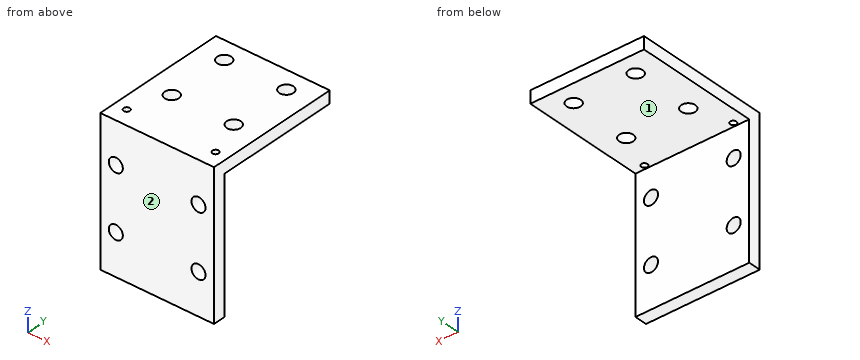
from build123d import *

# Parameters (mm, degrees)
SKETCH1_W                = 27.5
SKETCH1_H                = 3
BOSS_EXTRUDE1_DEPTH      = 35
SKETCH2_W                = 27.5
SKETCH2_H                = 3
BOSS_EXTRUDE2_DEPTH      = 40
M3_CLEARANCE_HOLE1_D     = 3.4
M3_CLEARANCE_HOLE1_DEPTH = 5
M3_CLEARANCE_HOLE1_TIP   = 1.021463052
SKETCH6_R                = 0.75
CUT_EXTRUDE1_DEPTH       = 10
M3_CLEARANCE_HOLE2_D     = 3.4
M3_CLEARANCE_HOLE2_DEPTH = 5
M3_CLEARANCE_HOLE2_TIP   = 1.021463052
SKETCH12_W               = 27.5
SKETCH12_H               = 10
CUT_EXTRUDE2_DEPTH       = 4


with BuildPart() as part:
    # Sketch1 → Boss-Extrude1 (new body)
    with BuildSketch(Plane.XY):
        Rectangle(SKETCH1_W, SKETCH1_H)
    extrude(amount=BOSS_EXTRUDE1_DEPTH)

    # Sketch2 → Boss-Extrude2 (add)
    with BuildSketch(Plane(origin=(0, 1.5, 0), x_dir=(1, 0, 0), z_dir=(0, 1, 0))):
        with Locations((0, -33.5)):
            Rectangle(SKETCH2_W, SKETCH2_H)
    extrude(amount=BOSS_EXTRUDE2_DEPTH)

    # M3 Clearance Hole1
    with Locations(Plane(origin=(0, 1.5, 0), x_dir=(1, 0, 0), z_dir=(0, 1, 0))):
        with Locations((-10, -10), (-10, -25), (10, -25), (10, -10)):
            Hole(M3_CLEARANCE_HOLE1_D / 2, depth=M3_CLEARANCE_HOLE1_DEPTH)
            with Locations((0, 0, -(M3_CLEARANCE_HOLE1_DEPTH + M3_CLEARANCE_HOLE1_TIP / 2))):  # 118° drill point
                Cone(0, M3_CLEARANCE_HOLE1_D / 2, M3_CLEARANCE_HOLE1_TIP, mode=Mode.SUBTRACT)

    # Sketch6 → Cut-Extrude1 (cut)
    with BuildSketch(Plane.XY.offset(35)):
        with Locations((-10.75, 2.5)):
            Circle(SKETCH6_R)
    cut_extrude1 = extrude(amount=-CUT_EXTRUDE1_DEPTH, mode=Mode.SUBTRACT)

    # M3 Clearance Hole2
    with Locations(Plane(origin=(0, 0, 32), x_dir=(-1, 0, 0), z_dir=(0, 0, -1))):
        with Locations((-7.5, 11.5), (7.5, 11.5), (7.5, 26.5), (-7.5, 26.5)):
            Hole(M3_CLEARANCE_HOLE2_D / 2, depth=M3_CLEARANCE_HOLE2_DEPTH)
            with Locations((0, 0, -(M3_CLEARANCE_HOLE2_DEPTH + M3_CLEARANCE_HOLE2_TIP / 2))):  # 118° drill point
                Cone(0, M3_CLEARANCE_HOLE2_D / 2, M3_CLEARANCE_HOLE2_TIP, mode=Mode.SUBTRACT)

    # Mirror1: Cut-Extrude1 across plane
    add(cut_extrude1.mirror(Plane(origin=(0, 0, 0), x_dir=(0, 0, 1), z_dir=(1, 0, 0))), mode=Mode.SUBTRACT)

    # Sketch12 → Cut-Extrude2 (cut, through all)
    with BuildSketch(Plane(origin=(0, 0, 32), x_dir=(-1, 0, 0), z_dir=(0, 0, -1))):
        with Locations((0, 36.5)):
            Rectangle(SKETCH12_W, SKETCH12_H)
    extrude(amount=-CUT_EXTRUDE2_DEPTH, mode=Mode.SUBTRACT)


solid = part.part
Geometry: final body of the model. Coordinates: model frame, mm. Face numbers are marked on the shaded views. A direction names the side the tool comes from. Give positions to 0.01 mm unless a question says otherwise; leave off trailing zeros. Write each loop counter-clockwise with the first axis right and the second up, starting at its lowest first coordinate (ties: lowest second). Pieces come first, ordered by that corner, then holes. Notation, with made-up numbers: M 84,18.5 L 140,18.5 A10 ccw 140,36.5 Z; hole C 52,51.5 d10. An arc over 180 degrees is marked long. Answer in a Markdown table with one row per item. Add a question column.
(1) Ray query, line 1 (X direction, y = -0.15, z = 25); line 2 (Y direction, x = 10.75, z = 33.65); line 3 (X direction, y = 27, z = 33). Return the intervals inside material, ascending.
(2) Section A-A on x = -7.5. Return loops of the section in (y, z), and give its area (3 significant figures).
(3) Section B-B on y = 2.5. Return loops of the section in (x, z), and give its area (3 significant figures).
(4) First-contact query: pin 1 (4 mm diameter, centred on x = -10, z = 25, fed in from -Y); pin 2 (2.5 mm diameter, centred on x = 7.5, y = 11.5, fed in from +Z); pin 3 (5.5 mm diameter, centred on x = 10, z = 25, fed in from +Y); pin 4 (1.7 mm diameter, centred on x = -10.75, y = 2.5, fed in from -Z). Flat tips, straight axial feed; report the tip coordinate or a pass-through.
(5) Section D-D on x = -10.75. Return loops of the section in (y, z).
(6) Reachability of the marked faces 1 and 2 from +Z, -Z, +X, -X, +Y, -Y: full face, straight path, thin tool, end or side. Return the list, or none.
(7) Section C-C on z = 10. Return loops of the section in (x, y), and give its area (3 significant figures).
Result set:
| question | item | result |
|---|---|---|
| 1 | line 1 | x = -13.75 to -11.7, -8.3 to 8.3, 11.7 to 13.75 |
| 1 | line 2 | y = -1.5 to 1.75, 3.25 to 31.5 |
| 1 | line 3 | x = -13.75 to -9.12, -5.88 to 5.88, 9.12 to 13.75 |
| 2 | outline | M -1.5,0 L 1.5,0 L 1.5,32 L 9.8,32 L 9.8,35 L -1.5,35 Z; M 13.2,32 L 24.8,32 L 24.8,35 L 13.2,35 Z; M 28.2,32 L 31.5,32 L 31.5,35 L 28.2,35 Z |
| 2 | area | 175 mm^2 |
| 3 | outline | M -13.75,32 L -11.5,32 L -11.5,35 L -13.75,35 Z; M -10,32 L 10,32 L 10,35 L -10,35 Z; M 11.5,32 L 13.75,32 L 13.75,35 L 11.5,35 Z |
| 3 | area | 73.5 mm^2 |
| 4 | pin 1 | stops at y = -1.5 |
| 4 | pin 2 | passes through |
| 4 | pin 3 | stops at y = 1.5 |
| 4 | pin 4 | stops at z = 32 |
| 5 | outline | M -1.5,0 L 1.5,0 L 1.5,8.47 L -1.5,8.47 Z; M -1.5,11.53 L 1.5,11.53 L 1.5,23.47 L -1.5,23.47 Z; M -1.5,26.53 L 1.5,26.53 L 1.5,32 L 1.75,32 L 1.75,35 L -1.5,35 Z; M 3.25,32 L 31.5,32 L 31.5,35 L 3.25,35 Z |
| 6 | face 1 | -Z, +X, -X, +Y |
| 6 | face 2 | +Z, -Z, +X, -X, -Y |
| 7 | outline | M -13.75,-1.5 L -11.7,-1.5 L -11.7,1.5 L -13.75,1.5 Z; M -8.3,-1.5 L 8.3,-1.5 L 8.3,1.5 L -8.3,1.5 Z; M 11.7,-1.5 L 13.75,-1.5 L 13.75,1.5 L 11.7,1.5 Z |
| 7 | area | 62.1 mm^2 |
